Here's the drawing with two shaded views (mm, measured from the low corner). I have some questions. A direction names the side the tool comes from. Give positions to 0.01 mm unless a question says otherwise; leave off trailing zeros. Write each loop counter-clockwise with the first axis right and the second up, starting at its lowest first coordinate (ties: lowest second). Pieces come first, ordered by that corner, then holes.
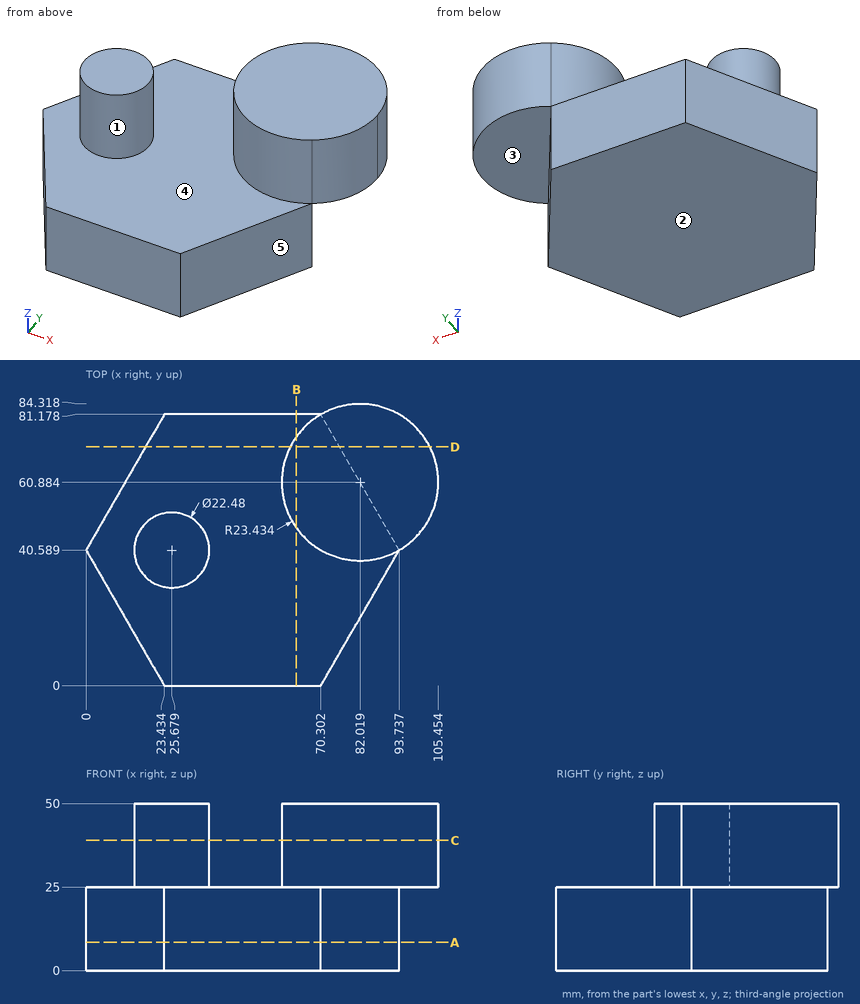
(1) For the marked faces 1 and 2, which set-ups out of +Z, -Z, +X, -X, +Y, -Y let a thin tool reach every point of the face, with its end or its side?
Returned:
face 1: +Z
face 2: -Z, +X, -X, +Y, -Y
(2) Imagine slicing it at B-B, the plane x = 63. Write out the boundary of the cut face in (y, z).
Returned:
outline: (0, 0) - (81.18, 0) - (81.18, 25) - (74.57, 25) - (74.57, 50) - (47.19, 50) - (47.19, 25) - (0, 25) - close
(3) Imagine slicing it at D-D, the plane y = 71.5. Write out the boundary of the cut face in (x, z).
Returned:
outline: (17.85, 0) - (75.89, 0) - (75.89, 25) - (102.91, 25) - (102.91, 50) - (61.13, 50) - (61.13, 25) - (17.85, 25) - close
(4) If we mould it in two halves opening along X, with no side actions, what happens to the marked faces 3, 4 and 5? For each: +X half, -X half, draft (parallel to the pull), parting line (faces both ways), or undercut.
Returned:
face 3: draft
face 4: undercut
face 5: +X half
(5) If I drill on L1, parallel to Z at x = 46.5, y = 39; L2, parallel to X at y = 43, z = 26.5 (1 decimal); L3, parallel to Z at x = 86, y = 56, over which ranges is the centre line in solid material (lowest first)?
Returned:
L1: z = 0 to 25
L2: x = 14.7 to 36.7, 66.9 to 97.2
L3: z = 25 to 50
(6) Will these pins go through, and if not, where does the flat tip stop? P1, Ø5, axis at x = 15.5, y = 9.5, coming from the +Z side; P2, Ø1, axis at x = 37.5, z = 19, coming from the +Y side; P3, Ø4, axis at y = 31, z = 38.5, coming from the -X side.
Returned:
P1: stops at z = 25
P2: stops at y = 81.18
P3: stops at x = 17.39
(7) Imagine slicing it at A-A, the plane z = 8.5. Write out the boundary of the cut face in (x, y) (1 decimal), plus the area to 3 significant figures.
Returned:
outline: (0, 40.6) - (23.4, 0) - (70.3, 0) - (93.7, 40.6) - (70.3, 81.2) - (23.4, 81.2) - close
area: 5,710 mm2
(8) Imagine slicing it at C-C, the plane z = 39. Write out the boundary of the cut face in (x, y) (1 decimal), plus the area to 3 significant figures.
Returned:
outline: circle Ø22.5 at (25.7, 40.6); (93.7, 40.6) arc R23.4 ccw to (105.5, 60.9) arc R23.4 ccw (long way) to start
area: 2,120 mm2
